The figure shows three views and two pictorial views of one solid part (mm, origin at its lowest corner). Answer the questions. Coordinates: 2 decimals unless noted, no trailing zeros. Order: outer loops, then holes, each group sorted by start corner. A loop starts at its lowest first (then second) coordinate and runs counter-clockwise, first axis right, second up. Notation, with made-up numbers: (57.25, -39.75) -> (75.25, -39.75) arc R21 cw to (75.25, -0.75) -> close; hole circle Ø8 at (-33.5, 38). An arc over 180 degrees is marked (long way). Return JSON: item names as keys, results as strings. Group by question number.
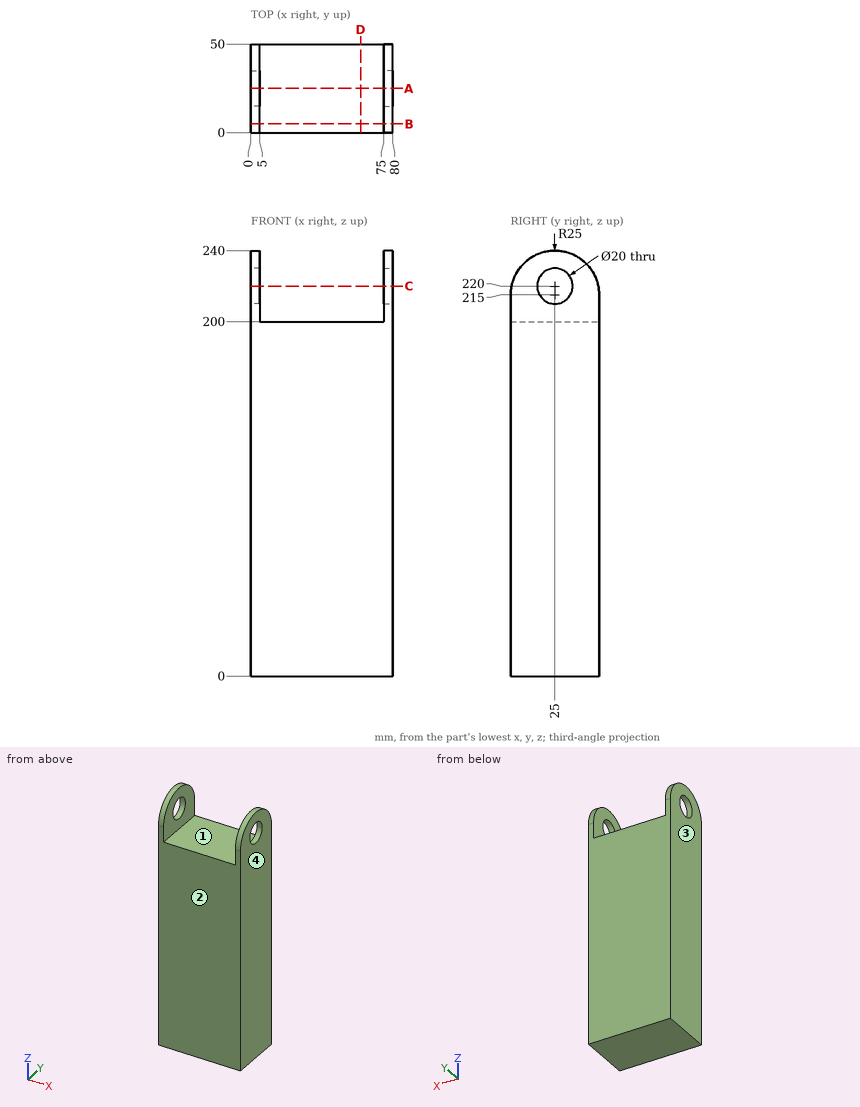
1. Given pin 1 (2 mm diameter, centred on x = 67.5, y = 40.5, fed in from +Z); pin 2 (12 mm diameter, centred on y = 25, z = 220, fed in from -X), each flat-ended and moving along its own axis, determine where each tip first touches the part or whether it passes through.
2. Find section A-A on y = 25. Determine the outline of the cut face in (x, z), and give its area (3 significant figures).
3. For a pull along X with two mould halves and no side action, classify the marked faces 1, 2, 3 and 4 as released by +X, released by -X, zero draft, split by the parting line, or undercut.
4. Find section C-C on z = 220. Determine the outline of the cut face in (x, y), and give its area (3 significant figures).
5. Straight lines are drawn through the part: L1, parallel to Z at x = 76.7, y = 25; L2, parallel to Z at x = 33.5, y = 24.5. For each, find the intervals that lie inside material, in ascending order.
6. Find section D-D on x = 62. Determine the outline of the cut face in (y, z).
7. Find section B-B on y = 5. Determine the outline of the cut face in (x, z).
Result:
{
 "1": {"pin 1": "z = 200", "pin 2": "through"},
 "2": {"outline": "(0, 0) -> (80, 0) -> (80, 210) -> (75, 210) -> (75, 200) -> (5, 200) -> (5, 210) -> (0, 210) -> close; (0, 230) -> (5, 230) -> (5, 240) -> (0, 240) -> close; (75, 230) -> (80, 230) -> (80, 240) -> (75, 240) -> close", "area": "16,200 mm^2"},
 "3": {"face 1": "undercut", "face 2": "zero draft", "face 3": "released by -X", "face 4": "released by +X"},
 "4": {"outline": "(0, 0.51) -> (5, 0.51) -> (5, 15) -> (0, 15) -> close; (0, 35) -> (5, 35) -> (5, 49.49) -> (0, 49.49) -> close; (75, 0.51) -> (80, 0.51) -> (80, 15) -> (75, 15) -> close; (75, 35) -> (80, 35) -> (80, 49.49) -> (75, 49.49) -> close", "area": "290 mm^2"},
 "5": {"L1": "0 to 210, 230 to 240", "L2": "0 to 200"},
 "6": {"outline": "(0, 0) -> (50, 0) -> (50, 200) -> (0, 200) -> close"},
 "7": {"outline": "(0, 0) -> (80, 0) -> (80, 230) -> (75, 230) -> (75, 200) -> (5, 200) -> (5, 230) -> (0, 230) -> close"}
}
